Design review of the part built by this model. Coordinates are the model's own, in mm. Face numbers are marked on the shaded views. Round coordinates to 2 decimals unless told otherwise and drop trailing zeros. Order: outer loops, then holes, each group sorted by start corner. A loop starts at its lowest first (then second) coordinate and runs counter-clockwise, first axis right, second up. Notation, with made-up numbers: M 23.25,-18.5 L 33.25,-18.5 A18 cw 33.25,-4.5 Z; hole C 65.5,35.5 d5. An arc over 180 degrees is marked long. Write each question's results on one line, items separated by ' | '. Start each with the question number.
Item 1: Wall thickness on line 1 (Y direction, x = 0, z = -5); line 2 (Y direction, x = -3.25, z = -6.25); line 3 (Y direction, x = -6, z = -2.25): over which ranges is each line inside the solid? List them lowest first. Write a range as [from, to].
Item 2: Take a section at B-B, the plane x = 0. Write out the cut boundary in (y, z).
Item 3: Clearance check with flat-ended pins moving along their axes: pin 1 (4 mm diameter, centred on x = -5, z = -2, fed in from +Y); pin 2 (5 mm diameter, centred on x = -0.5, y = -4, fed in from -Z); pin 3 (1 mm diameter, centred on y = -5.5, z = -2, fed in from -X). State where each tip first meets the part, or that it passes through.
Item 4: The part is to be moulded in two halves that separate along Y. For the marked faces 1, 2 and 3, say which applies: +Y half, -Y half, draft (parallel to the pull), parting line (faces both ways), or undercut.
Item 5: Take a section at C-C, the plane z = -1.75. Write out the cut boundary in (x, y).
Item 6: Take a section at A-A, the plane y = -2.5. Write out the cut boundary in (x, z).
Autodesk Inventor part; units mm, degrees
ref_plane "YZ Plane" through (0, 0, 0) normal (1, 0, 0) x (0, 1, 0)
ref_plane "XZ Plane" through (0, 0, 0) normal (0, 1, 0) x (-1, 0, 0)
ref_plane "XY Plane" through (0, 0, 0) normal (0, 0, 1) x (1, 0, 0)
sketch "Skizze1" plane through (0, 0, 0) normal (0, 0, 1) x (1, 0, 0)
  circle A0 centre (0, -2.5) radius 5
  circle A1 centre (0, -2.5) radius 2.5
  circle A2 centre (0, -2.5) radius 6.5
  point P0 (0, 0)
  dimension "d0" = 13
extrude "Extrusion1" add sketch "Skizze1" against normal blind 7 contours A2
thread "Gewinde1"
sketch "Skizze2" plane through (0, -2.5, 0) normal (0, 0, 1) x (1, 0, 0)
  circle A0 centre (0, 0) radius 6.5
  point P0 (0, 2.5)
extrude "Extrusion2" add sketch "Skizze2" along normal blind 2
fillet "Rundung1" radius 2 1 edges at (-6.5, -2.5, 2)
properties part number "Mutter"
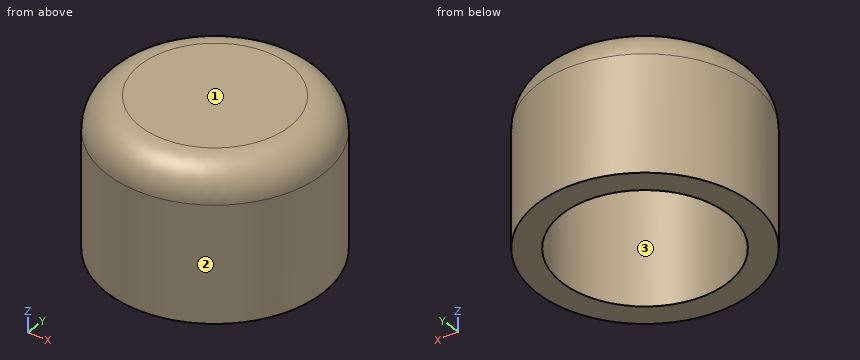
Results list:
1) line 1: [-9, -7.5], [2.5, 4] | line 2: [-8.13, -6.3], [1.3, 3.13] | line 3: [-5, 0]
2) outline: M -9,-7 L -7.5,-7 L -7.5,0 L 2.5,0 L 2.5,-7 L 4,-7 L 4,0 A2 ccw 2,2 L -7,2 A2 ccw -9,0 Z
3) pin 1: y = 3.27 | pin 2: z = 0 | pin 3: x = -6
4) face 1: draft | face 2: parting line | face 3: undercut
5) outline: C 0,-2.5 d13; hole C 0,-2.5 d10
6) outline: M -6.5,-7 L -5,-7 L -5,0 L 5,0 L 5,-7 L 6.5,-7 L 6.5,0 A2 ccw 4.5,2 L -4.5,2 A2 ccw -6.5,0 Z
